Could you check a few things on this model? Use its own coordinates, in mm. A direction names the side the tool comes from. Give positions to 0.01 mm unless a question says otherwise; leave off trailing zeros. Loops run counter-clockwise (first coordinate to the right, second up) from the corner with the lowest first, then second, coordinate; pieces in that order, holes last. Notation, with made-up numbers: (55, 48.5) -> (71, 48.5) arc R10 cw to (71, 56.5) -> close; hole circle Ø10 at (29.5, 46.25). An arc over 180 degrees is marked (long way). Write item = value, one per line. Start each with the question number.
1) I want a section at A-A (z = 19.75). List the corners of the cut face in (x, y) for me.
2) On a 3-axis mill with a long thin cutter (end or side, diameter ignored), from which of +Z, -Z, +X, -X, +Y, -Y can I reach the whole of each face in a straight line? I mean faces 5 (the face through (-6.03, 35.28, 10.1)), 6 (the face through (7.5, -50, 15)), 7 (the face through (12.056, 15.338, 3.475)), 8 (the face through (-4, -77, 13)), 9 (the face through (-5, -48.5, 2)). Say none if no direction works.
3) If we mould it in two halves opening along Z, with no side actions, what happens to faces 1 (the face through (-17.5, -50, 15)), 2 (the face through (12, 23.25, 8)), 3 (the face through (-8, 14, 16)), 4 (the face through (-12.06, 21.78, 3.87))? For each: +Z half, -Z half, draft (parallel to the pull), parting line (faces both ways), or undercut.
4) I'm going to push flat-ended pins straight in: pin 1 Ø8 at (y, z) = (33, 8) entering from +X; pin 2 Ø13 at (y, z) = (35.5, 8.5) entering from -X; pin 3 Ø2 at (x, y) = (-14.5, -6.5) entering from +Z. Where does each tip first touch, or does it pass through?
5) I want a section at B-B (y = 51). List the corners of the cut face in (x, z) for me.
6) I need wall thicknesses on probe 1 along Z at (x, y) = (-6, 33); probe 2 along Y at (x, z) = (0, 11.25); probe 3 along Y at (x, z) = (-5, 20.25). Which ranges of each line are inside material? Lowest first, please. Write a range as from..to.
from build123d import *

# Parameters (mm, degrees)
SKETCH_1_R               = 11.5
SKETCH_1_W               = 25
SKETCH_1_H               = 45.5
EXTRUDE_1_DEPTH          = 16
SKETCH_2_R               = 3.1
CUT_EXTRUDE_1_DEPTH      = 120.143820654
SKETCH_2_2_R             = 5.6
SKETCH_2_2_R_2           = 3.1
CUT_EXTRUDE_1_2_DEPTH    = 8
CUT_EXTRUDE_2_DEPTH      = 108.64408948
CUT_EXTRUDE_2_DEPTH_BACK = 108.64408948
SKETCH_3_W               = 8
SKETCH_3_H               = 51
CUT_EXTRUDE_2_2_DEPTH    = 8
CHAMFER_1_SIZE           = 1.695682666
CHAMFER_1_SIZE_2         = 1
SKETCH_1_2_W             = 25
SKETCH_1_2_H             = 45.5
EXTRUDE_2_DEPTH          = 4
SKETCH_6_R               = 3.25
CUT_EXTRUDE_3_DEPTH      = 108.122593322
SKETCH_7_W               = 39.5
SKETCH_7_H               = 56.25
SKETCH_7_W_2             = 25
SKETCH_7_H_2             = 45.5
SKETCH_7_W_3             = 37
EXTRUDE_3_DEPTH          = 10
FILLET_1_R               = 2
CHAMFER_2_SIZE           = 1
CHAMFER_3_SIZE           = 25
CUT_EXTRUDE_4_DEPTH      = 108.64408948
CUT_EXTRUDE_4_DEPTH_BACK = 108.64408948
SKETCH_8_W               = 71.361850602
SKETCH_8_H               = 94.902741324
FILLET_2_R               = 2


with BuildPart() as part:
    # 草图1 → 凸台-拉伸1 (new body)
    with BuildSketch(Plane.XY):
        Polygon((16, 66), (-16, 66), (-16, -15), (-23.5, -15), (-23.5, -77), (13.5, -77), (73.5, -77), (73.5, -15), (16, -15), align=None)
        with Locations((0, 51)):
            Circle(SKETCH_1_R, mode=Mode.SUBTRACT)
        Circle(SKETCH_1_R, mode=Mode.SUBTRACT)
        with Locations((-5, -49.5)):
            Rectangle(SKETCH_1_W, SKETCH_1_H, mode=Mode.SUBTRACT)
        with Locations((55, -49.5)):
            Rectangle(SKETCH_1_W, SKETCH_1_H, mode=Mode.SUBTRACT)
    extrude(amount=EXTRUDE_1_DEPTH)

    # 草图2 → Cut-Extrude 1 (cut, through all)
    with BuildSketch(Plane.ZY.offset(16)):
        with Locations(Location((8, 33, 0), (0, 0, 270))):
            Circle(SKETCH_2_R)
        with Locations(Location((8, 18, 0), (0, 0, 270))):
            Circle(SKETCH_2_R)
    extrude(amount=-CUT_EXTRUDE_1_DEPTH, mode=Mode.SUBTRACT)

    # 草图2<2> → Cut-Extrude 1 2 (cut)
    # profile 1 of 2: a face of its own
    with BuildSketch(Plane.ZY.offset(16)):
        with Locations((8, 33)):
            Circle(SKETCH_2_2_R)
        with Locations((8, 33)):
            Circle(SKETCH_2_2_R_2, mode=Mode.SUBTRACT)
    # profile 2 of 2: a face of its own
    with BuildSketch(Plane.ZY.offset(16)):
        with Locations((8, 18)):
            Circle(SKETCH_2_2_R)
        with Locations((8, 18)):
            Circle(SKETCH_2_2_R_2, mode=Mode.SUBTRACT)
    extrude(amount=-CUT_EXTRUDE_1_2_DEPTH, mode=Mode.SUBTRACT)

    # 草图3 → Cut-Extrude 2 (cut, two sides: drawn at the far end of the back side and taken through both)
    with BuildSketch(Plane.XY.offset(16).offset(-CUT_EXTRUDE_2_DEPTH_BACK)):
        with Locations((0, 25.5)):
            Rectangle(SKETCH_3_W, SKETCH_3_H)
    extrude(amount=CUT_EXTRUDE_2_DEPTH + CUT_EXTRUDE_2_DEPTH_BACK, mode=Mode.SUBTRACT)

    # 草图4 → Cut-Extrude 2 2 (cut)
    with BuildSketch(Plane(origin=(16, 0, 0), x_dir=(0, 0, -1), z_dir=(1, 0, 0))):
        Polygon((-1.937822174, 33), (-4.968911087, 38.25), (-11.031088913, 38.25), (-14.062177826, 33), (-11.031088913, 27.75), (-4.968911087, 27.75), align=None)
        Polygon((-1.937822174, 18), (-4.968911087, 23.25), (-11.031088913, 23.25), (-14.062177826, 18), (-11.031088913, 12.75), (-4.968911087, 12.75), align=None)
    extrude(amount=-CUT_EXTRUDE_2_2_DEPTH, mode=Mode.SUBTRACT)

    # 倒角1
    # the kernel refuses this chamfer: 1.695682666, 1 mm, written as the material it takes off along each edge
    with BuildSketch(Plane(origin=(-4, 40.218070674, 20.393897044), x_dir=(0, -1, 0), z_dir=(0, 0, -1))) as chamfer_1_piece_1:
        with BuildLine():
            Line((CHAMFER_1_SIZE, 0), (-0.409315042, 0.965770122))
            ThreePointArc((-0.409315042, 0.965770122), (-0.203470382, 0.51067693), (0, 0))
            Line((0, 0), (CHAMFER_1_SIZE, 0))
        make_face()
    extrude(amount=24.787794087, mode=Mode.SUBTRACT)
    with BuildSketch(Plane(origin=(-4, 10.781929326, 20.393897044), x_dir=(0, 1, 0), z_dir=(0, 0, -1))) as chamfer_1_piece_2:
        with BuildLine():
            Line((CHAMFER_1_SIZE, 0), (-0.409315042, -0.965770122))
            ThreePointArc((-0.409315042, -0.965770122), (-0.203470382, -0.51067693), (0, 0))
            Line((0, 0), (CHAMFER_1_SIZE, 0))
        make_face()
    extrude(amount=24.787794087, mode=Mode.SUBTRACT)
    with BuildSketch(Plane(origin=(4, 40.218070674, 21.505815426), x_dir=(0.9011630930702207, 0.4334801952663038, 0), z_dir=(0, 0, -1))) as chamfer_1_piece_3:
        with BuildLine():
            Line((2.138200915, 0), (-CHAMFER_1_SIZE_2 * 0.433480195266, CHAMFER_1_SIZE_2 * 0.90116309307))
            Line((-CHAMFER_1_SIZE_2 * 0.433480195266, CHAMFER_1_SIZE_2 * 0.90116309307), (0, 0))
            ThreePointArc((0, 0), (1.101276568, 0.049757425), (2.138200915, 0))
        make_face()
    extrude(amount=27.011630851, mode=Mode.SUBTRACT)
    with BuildSketch(Plane(origin=(4, 10.781929326, 21.505815426), x_dir=(0, 1, 0), z_dir=(0, 0, -1))) as chamfer_1_piece_4:
        with BuildLine():
            Line((CHAMFER_1_SIZE_2, 0), (-0.92686775, 1.92686775))
            ThreePointArc((-0.92686775, 1.92686775), (-0.432542027, 1.013998656), (0, 0))
            Line((0, 0), (CHAMFER_1_SIZE_2, 0))
        make_face()
    extrude(amount=27.011630851, mode=Mode.SUBTRACT)

    # 草图1<2> → 凸台-拉伸2 (add)
    with BuildSketch(Plane.XY):
        with Locations((-5, -49.5)):
            Rectangle(SKETCH_1_2_W, SKETCH_1_2_H)
        with Locations((55, -49.5)):
            Rectangle(SKETCH_1_2_W, SKETCH_1_2_H)
    extrude(amount=EXTRUDE_2_DEPTH)

    # 草图6 → 切除-拉伸3 (cut, through all)
    with BuildSketch(Plane.XY.offset(4)):
        with Locations((-5, -37)):
            Circle(SKETCH_6_R)
        with Locations((55, -37)):
            Circle(SKETCH_6_R)
        Polygon((-16.25, -54.9), (-14.5, -54.9), (-14.5, -69.9), (4.5, -69.9), (4.5, -54.9), (6.25, -54.9), (6.25, -48.5), (-16.25, -48.5), align=None)
        Polygon((45.5, -54.9), (43.75, -54.9), (43.75, -48.5), (66.25, -48.5), (66.25, -54.9), (64.5, -54.9), (64.5, -69.9), (45.5, -69.9), align=None)
    extrude(amount=-CUT_EXTRUDE_3_DEPTH, mode=Mode.SUBTRACT)

    # 草图7 → 凸台-拉伸3 (add)
    # profile 1 of 2: a face of its own
    with BuildSketch(Plane.XY.offset(16)):
        with Locations((-3.75, -48.875)):
            Rectangle(SKETCH_7_W, SKETCH_7_H)
        with Locations((-5, -49.5)):
            Rectangle(SKETCH_7_W_2, SKETCH_7_H_2, mode=Mode.SUBTRACT)
    # profile 2 of 2: a face of its own
    with BuildSketch(Plane.XY.offset(16)):
        with Locations((55, -48.875)):
            Rectangle(SKETCH_7_W_3, SKETCH_7_H)
        with Locations((55, -49.5)):
            Rectangle(SKETCH_7_W_2, SKETCH_7_H_2, mode=Mode.SUBTRACT)
    extrude(amount=EXTRUDE_3_DEPTH)

    # 圆角1
    fillet_1_edges = [part.edges().sort_by_distance(p)[0] for p in [
        (-16, 66, 8),
        (16, 66, 8),
        (73.5, -15, 8),
        (73.5, -77, 13),
        (-23.5, -77, 13),
        (-23.5, -15, 8),
        (-16, -15, 8),
    ]]
    fillet(fillet_1_edges, radius=FILLET_1_R)

    # 倒角2
    # the kernel refuses this chamfer: 1 mm, written as the material it takes off along each edge
    with BuildSketch(Plane(origin=(-4, 9.905929004, 16), x_dir=(-1, 0, 0), z_dir=(0, 1, 0))) as chamfer_2_piece_1:
        Polygon((CHAMFER_2_SIZE, 0), (0, -CHAMFER_2_SIZE), (0, 0), align=None)
    extrude(amount=31.188141991, mode=Mode.SUBTRACT)
    with BuildSketch(Plane(origin=(-4, 9.905929004, 0), x_dir=(-1, 0, 0), z_dir=(0, 1, 0))) as chamfer_2_piece_2:
        Polygon((CHAMFER_2_SIZE, 0), (0, CHAMFER_2_SIZE), (0, 0), align=None)
    extrude(amount=31.188141991, mode=Mode.SUBTRACT)
    with BuildSketch(Plane(origin=(0, 0, 16), x_dir=(0.15887239859298968, 0.9872991243616649, 0), z_dir=(-0.9872991243616649, 0.15887239859298968, 0))) as chamfer_2_piece_3:
        Polygon((11.5 + CHAMFER_2_SIZE, 0), (11.5, CHAMFER_2_SIZE), (11.5, 0), align=None)
    revolve(axis=Axis((0, 0, 16), (0, 0, -1)), revolution_arc=338.147720881, mode=Mode.SUBTRACT)
    with BuildSketch(Plane(origin=(0, 0, 0), x_dir=(-0.22003054145636358, 0.9754929834839509, 0), z_dir=(0.9754929834839509, 0.22003054145636358, 0))) as chamfer_2_piece_4:
        Polygon((11.5 + CHAMFER_2_SIZE, 0), (11.5, CHAMFER_2_SIZE), (11.5, 0), align=None)
    revolve(axis=Axis((0, 0, 0), (0, 0, 1)), revolution_arc=338.147720881, mode=Mode.SUBTRACT)
    with BuildSketch(Plane(origin=(4, 41.789753662, 16), x_dir=(1, 0, 0), z_dir=(0, -1, 0))) as chamfer_2_piece_5:
        Polygon((CHAMFER_2_SIZE, 0), (0, -CHAMFER_2_SIZE), (0, 0), align=None)
    extrude(amount=32.579507323, mode=Mode.SUBTRACT)
    with BuildSketch(Plane(origin=(4, 41.789753662, 0), x_dir=(1, 0, 0), z_dir=(0, -1, 0))) as chamfer_2_piece_6:
        Polygon((CHAMFER_2_SIZE, 0), (0, CHAMFER_2_SIZE), (0, 0), align=None)
    extrude(amount=32.579507323, mode=Mode.SUBTRACT)
    with BuildSketch(Plane(origin=(0, 51, 0), x_dir=(0.15887239859295355, -0.9872991243616707, 0), z_dir=(-0.9872991243616707, -0.15887239859295355, 0))) as chamfer_2_piece_7:
        Polygon((11.5 + CHAMFER_2_SIZE, 0), (11.5, CHAMFER_2_SIZE), (11.5, 0), align=None)
    revolve(axis=Axis((0, 51, 0), (0, 0, 1)), revolution_arc=338.147720881, mode=Mode.SUBTRACT)
    with BuildSketch(Plane(origin=(0, 51, 16), x_dir=(-0.2200305414563642, -0.9754929834839506, 0), z_dir=(0.9754929834839506, -0.2200305414563642, 0))) as chamfer_2_piece_8:
        Polygon((11.5 + CHAMFER_2_SIZE, 0), (11.5, CHAMFER_2_SIZE), (11.5, 0), align=None)
    revolve(axis=Axis((0, 51, 16), (0, 0, -1)), revolution_arc=338.147720881, mode=Mode.SUBTRACT)

    # 倒角3
    chamfer_3_edges = [part.edges().sort_by_distance(p)[0] for p in [
        (16, -15, 8),
    ]]
    chamfer(chamfer_3_edges, length=CHAMFER_3_SIZE)

    # 草图8 → 切除-拉伸4 (cut, two sides: drawn at the far end of the back side and taken through both)
    with BuildSketch(Plane.XY.offset(16).offset(-CUT_EXTRUDE_4_DEPTH_BACK)):
        with Locations((51.680925301, -37.451370662)):
            Rectangle(SKETCH_8_W, SKETCH_8_H)
    extrude(amount=CUT_EXTRUDE_4_DEPTH + CUT_EXTRUDE_4_DEPTH_BACK, mode=Mode.SUBTRACT)

    # 圆角2
    fillet_2_edges = [part.edges().sort_by_distance(p)[0] for p in [
        (16, -77, 13),
    ]]
    fillet(fillet_2_edges, radius=FILLET_2_R)


solid = part.part
Answer list:
q1.outline = (-23.5, -75) arc R2 ccw to (-21.5, -77) -> (14, -77) arc R2 ccw to (16, -75) -> (16, -20.75) -> (-23.5, -20.75) -> close; hole (-17.5, -72.25) -> (7.5, -72.25) -> (7.5, -26.75) -> (-17.5, -26.75) -> close
q2.face_5 = +X, -X
q2.face_6 = +Z
q2.face_7 = +X
q2.face_8 = +Z, -Z, +X, -X, -Y
q2.face_9 = +Z, -Z
q3.face_1 = draft
q3.face_2 = undercut
q3.face_3 = +Z half
q3.face_4 = undercut
q4.pin_1 = 8
q4.pin_2 = -16
q4.pin_3 = 16
q5.outline = (-16, 0) -> (-12.5, 0) -> (-11.5, 1) -> (-11.5, 15) -> (-12.5, 16) -> (-16, 16) -> close; (11.5, 1) -> (12.5, 0) -> (16, 0) -> (16, 16) -> (12.5, 16) -> (11.5, 15) -> close
q6.probe_1 = 0..4.9, 11.1..16
q6.probe_2 = -77..-72.25, -26.75..-11.5, 62.5..66
q6.probe_3 = -77..-72.25, -26.75..-20.75
